Part model, mm, in its own coordinate system. Coordinates: 2 decimals unless noted, no trailing zeros. Loops run counter-clockwise (first coordinate to the right, second up) from the corner with the lowest first, then second, coordinate; pieces in that order, holes last. Notation, with made-up numbers: M -37,70 L -27,70 A30 cw -27,102 Z; hole C 38.25,7.25 d10. An arc over 180 degrees is marked long. Use a Markdown table: item, result. Add a question column.
1) Band-saw the part on C-C (z = -28). List the corners of the cut face in (x, y).
2) Band-saw the part on A-A (x = 0). List the corners of the cut face in (y, z).
3) Band-saw the part on B-B (y = 19.5). List the corners of the cut face in (x, z), plus the area to 3 significant figures.
4) Pin check, flat tips, straight feed: pin 1 Ø2 at (x, z) = (11.5, 4.5) entering from +Y; pin 2 Ø1.8 at (x, z) = (37.45, -56.76) entering from +Y. Stop position of each tip, or through.
5) Pull direction X, two halves, no side cores. Call faces 1 (the cylindrical face through (-1.084, -2.465, 28.936)), 2 (the flat face through (17.776, 17.325, -90.417)), 3 (the flat face through (13.03, 17.25, -92)): released by +X, released by -X, zero draft, split by the parting line, or undercut.
6) Wall check: probe 1 along Z at (x, y) = (0, -0.95); probe 2 along X at (y, z) = (-1.5, 38); probe 3 along Y at (x, z) = (4.5, 27.5). Give the ranges that are in metal, low to high. Write a range as from..to.
from build123d import *

# Parameters (mm, degrees)
F0_R     = 5
F0_R_2   = 1.5
F1_DEPTH = 5
F2_DEPTH = 35
F3_R     = 4.99999


# Not quite as in the source:
# - a fillet or chamfer is up to 0.001 mm smaller than in the source, because OpenCascade refuses the exact size


with BuildPart() as f1:
    # F0 (on Front) → F1 (new body)
    with BuildSketch(Plane.XZ):
        with BuildLine():
            ThreePointArc((14.7291057085, 20.287369527), (18.6357467541, 26.5570015397), (20, 33.8170940264))
            ThreePointArc((20, 33.8170940264), (-16.154238453, 45.6086409989), (6.0959419995, 14.7687478741))
            ThreePointArc((6.0959419995, 14.7687478741), (10.7719287617, 16.9658166044), (14.7291057085, 20.287369527))
        make_face()
        with Locations((0, 33.8170940264)):
            Circle(F0_R, mode=Mode.SUBTRACT)
        with BuildLine():
            ThreePointArc((14.7291057085, 20.287369527), (10.7719287617, 16.9658166044), (6.0959419995, 14.7687478741))
            Line((6.0959419995, 14.7687478741), (32.0687023036, -56.5908245822))
            Line((32.0687023036, -56.5908245822), (32.4609528428, -56.4480570615))
            ThreePointArc((32.4609528428, -56.4480570615), (36.7371185385, -51.8113638587), (42.1496687351, -55.0500082175))
            Line((42.1496687351, -55.0500082175), (14.7291057085, 20.287369527))
        make_face()
        with BuildLine():
            Line((32.4609528428, -56.4480570615), (32.0687023036, -56.5908245822))
            Line((32.0687023036, -56.5908245822), (32.5817325186, -58.0003635134))
            Line((32.5817325186, -58.0003635134), (32.7527425708, -58.4702097705))
            ThreePointArc((32.7527425708, -58.4702097705), (32.5024604285, -57.4741961437), (32.4609528428, -56.4480570615))
        make_face()
        with BuildLine():
            ThreePointArc((33.8290334161, -60.2068275447), (33.2012405538, -59.3940787929), (32.7527425708, -58.4702097705))
            Line((32.7527425708, -58.4702097705), (33.4367828769, -60.3495950653))
            Line((33.4367828769, -60.3495950653), (33.8290334161, -60.2068275447))
        make_face()
        with BuildLine():
            ThreePointArc((42.4512056942, -56.7601091071), (42.3752444432, -55.8918681281), (42.1496687351, -55.0500082175))
            ThreePointArc((42.1496687351, -55.0500082175), (36.7371185385, -51.8113638587), (32.4609528428, -56.4480570615))
            ThreePointArc((32.4609528428, -56.4480570615), (32.5024604285, -57.4741961437), (32.7527425708, -58.4702097705))
            ThreePointArc((32.7527425708, -58.4702097705), (33.2012405538, -59.3940787929), (33.8290334161, -60.2068275447))
            ThreePointArc((33.8290334161, -60.2068275447), (39.3071607865, -61.4028917528), (42.4512056942, -56.7601091071))
        make_face()
        with Locations((37.4512056942, -56.7601091071)):
            Circle(F0_R_2, mode=Mode.SUBTRACT)
        with BuildLine():
            Line((42.3206788698, -55.5198547009), (42.1496687351, -55.0500082175))
            ThreePointArc((42.1496687351, -55.0500082175), (42.3752444432, -55.8918681281), (42.4512056942, -56.7601091071))
            ThreePointArc((42.4512056942, -56.7601091071), (39.3071607865, -61.4028917528), (33.8290334161, -60.2068275447))
            Line((33.8290334161, -60.2068275447), (33.4367828769, -60.3495950653))
            Line((33.4367828769, -60.3495950653), (33.6077929485, -60.8194413757))
            Line((33.6077929485, -60.8194413757), (39.5341938332, -77.1020939848))
            Line((39.5341938332, -77.1020939848), (42.9543952664, -86.4990201927))
            Line((42.9543952664, -86.4990201927), (52.3513214743, -83.0788187594))
            Line((52.3513214743, -83.0788187594), (42.3206788698, -55.5198547009))
        make_face()
        Polygon((19.4620797468, -95.0495237758), (42.9543952664, -86.4990201927), (39.5341938332, -77.1020939848), (16.0418783135, -85.652597568), align=None)
        Polygon((14.7636166428, -96.7596244924), (19.4620797468, -95.0495237758), (16.0418783135, -85.652597568), (11.3434152096, -87.3626982846), align=None)
    extrude(amount=F1_DEPTH)

    # F0 (on Front) → F2 (join)
    with BuildSketch(Plane.XZ):
        Polygon((14.7636166428, -96.7596244924), (19.4620797468, -95.0495237758), (16.0418783135, -85.652597568), (11.3434152096, -87.3626982846), align=None)
    extrude(amount=-F2_DEPTH)

    # F3 (radius 5 in the source; OpenCascade refuses exactly that, so slightly less here)
    f3_edges = [f1.edges().sort_by_distance(p)[0] for p in [
        (6.095942, -2.5, 14.768748),
        (14.729106, -2.5, 20.28737),
        (52.351321, -2.5, -83.078819),
        (17.751979, 0, -90.351061),
        (13.053516, -5, -92.061161),
        (39.534194, -2.5, -77.102094),
        (17.751979, 35, -90.351061),
    ]]
    fillet(f3_edges, radius=F3_R)


solid = f1.part
Entries:
| question | item | result |
|---|---|---|
| 1 | outline | M 21.66,-5 L 32.3,-5 L 32.3,0 L 21.66,0 Z |
| 2 | outline | M -5,13.82 L 0,13.82 L 0,28.82 L -5,28.82 Z; M -5,38.82 L 0,38.82 L 0,53.82 L -5,53.82 Z |
| 3 | outline | M 11.34,-87.36 L 14.76,-96.76 L 19.46,-95.05 L 16.04,-85.65 Z |
| 3 | area | 50.0 mm2 |
| 4 | pin 1 | y = 0 |
| 4 | pin 2 | through |
| 5 | face 1 | undercut |
| 5 | face 2 | released by +X |
| 5 | face 3 | released by -X |
| 6 | probe 1 | 13.82..28.82, 38.82..53.82 |
| 6 | probe 2 | -19.56..-2.74, 2.74..19.56 |
| 6 | probe 3 | -5..0 |
